Autodesk Inventor part; units mm, degrees
ref_plane "YZ Plane" through (0, 0, 0) normal (1, 0, 0) x (0, 1, 0)
ref_plane "XZ Plane" through (0, 0, 0) normal (0, 1, 0) x (-1, 0, 0)
ref_plane "XY Plane" through (0, 0, 0) normal (0, 0, 1) x (1, 0, 0)
sketch "Sketch1" plane through (0, 0, 0) normal (0, 0, 1) x (1, 0, 0)
  line L0 (-137.16, 0) -> (22.86, 0)
  line L1 (0, -160.02) -> (0, 160.02)
  arc A0 (0, 114.3) -> (0, -114.3) centre (0, 0) ccw
  arc A1 (0, 111.125) -> (0, -111.125) centre (0, 0) ccw
  line L2 (0, 111.125) -> (0, 114.3)
  line L3 (0, -114.3) -> (0, -111.125)
  dimension "d6" = 3.175
  dimension "d7" = 228.6
revolve "Revolution1" add sketch "Sketch1" angle 180 about axis through (0, -10, 0) along (0, 1, 0) contours A0 L1 A1 L0 | L0 A1 L1 A0
sketch "Sketch2" plane through (0, 0, 0) normal (0, 0, -1) x (-1, 0, 0)
  circle A0 centre (0, 0) radius 114.3
  line L0 (-6.35, 114.1235) -> (-6.35, 6.4165)
  line L1 (-6.35, 6.4165) -> (-114.1198, 6.4165)
  line L2 (160.02, 0) -> (-160.02, 0)
  line L3 (0, -160.02) -> (0, 160.02)
  line L4 (-114.3, 0.0665) -> (114.3, 0.0665) construction
  dimension "d2" = 6.35
  dimension "d3" = 6.35
extrude "Extrusion1" cut sketch "Sketch2" against normal through all contours L0 L1 A0
mirror "Mirror1" about plane through (0, 0, 0) normal (0, 1, 0) of "Extrusion1"
mirror "Mirror2" about plane through (0, 0, 0) normal (1, 0, 0) of "Extrusion1", "Mirror1"
properties part number "shell model"
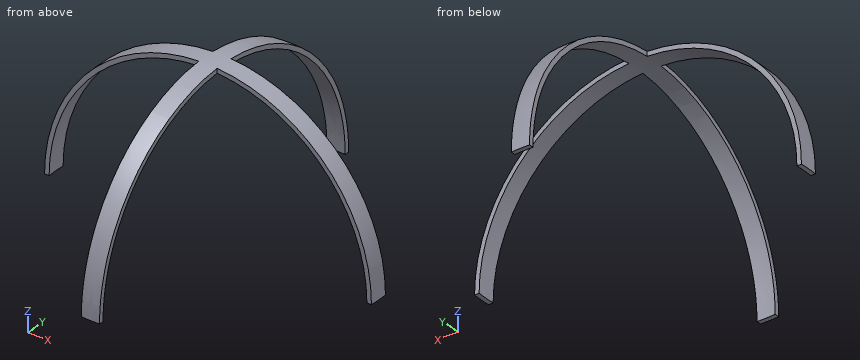
CAD build for the part. Positions are in the model's coordinates, mm. Round coordinates to 2 decimals unless told otherwise and drop trailing zeros. Write each loop counter-clockwise with the first axis right and the second up, starting at its lowest first coordinate (ties: lowest second). Pieces come first, ordered by that corner, then holes. Notation, with made-up numbers: (73, 44.25) -> (123, 44.25) arc R31 cw to (123, 73.25) -> close; hole circle Ø10 at (68.5, 52). An arc over 180 degrees is marked (long way). Answer in a Markdown table with one row per item. Add a question column.
Item 1: Saw through at C-C, the plane x = -53. Write the cut outline in (y, z).
Item 2: Drop flat-ended pins along their axis: pin 1 Ø10 at (y, z) = (-10.5, 19) entering from +X; pin 2 Ø8 at (x, y) = (5.5, -67.5) entering from -Z. Give the stop position or say it passes through.
Item 3: Drill centre lines: line 1 (X direction, y = 76.5, z = 81.5); line 2 (Z direction, x = 5, y = 20.5); line 3 (Z direction, x = 24.5, y = -5.5). Where is each one in solid material? Low to high. Write a range as from..to.
Item 4: Saw through at D-D, the plane y = 98. Write the cut outline in (x, z).
Item 5: Saw through at B-B, the plane z = 92.5. Write the cut outline in (x, y).
Item 6: Saw through at A-A, the plane z = 79. Write the cut outline in (x, y), then the cut area to 3 significant figures.
Findings below:
| question | item | result |
|---|---|---|
| 1 | outline | (-6.42, 97.46) arc R97.67 cw to (6.42, 97.46) -> (6.42, 101.07) arc R101.27 ccw to (-6.42, 101.07) -> close |
| 2 | pin 1 | stops at x = 112.98 |
| 2 | pin 2 | stops at z = 84.88 |
| 3 | line 1 | x = -6.35..6.35 |
| 3 | line 2 | z = 109.1..112.34 |
| 3 | line 3 | z = 108.25..111.51 |
| 4 | outline | (-6.35, 52) arc R52.39 cw to (6.35, 52) -> (6.35, 58.48) arc R58.83 ccw to (-6.35, 58.48) -> close |
| 5 | outline | (-66.84, -6.42) -> (-61.25, -6.42) arc R61.58 cw to (-61.25, 6.42) -> (-66.84, 6.42) arc R67.14 ccw to start; (-6.35, -66.84) arc R67.14 ccw to (6.35, -66.84) -> (6.35, -61.26) arc R61.58 cw to (-6.35, -61.26) -> close; (-6.35, 61.26) arc R61.58 cw to (6.35, 61.26) -> (6.35, 66.84) arc R67.14 ccw to (-6.35, 66.84) -> close; (61.25, -6.42) -> (66.84, -6.42) arc R67.14 ccw to (66.84, 6.42) -> (61.25, 6.42) arc R61.58 cw to start |
| 6 | outline | (-82.35, -6.42) -> (-77.89, -6.42) arc R78.15 cw to (-77.89, 6.42) -> (-82.35, 6.42) arc R82.6 ccw to start; (-6.35, -82.36) arc R82.6 ccw to (6.35, -82.36) -> (6.35, -77.89) arc R78.15 cw to (-6.35, -77.89) -> close; (-6.35, 77.89) arc R78.15 cw to (6.35, 77.89) -> (6.35, 82.36) arc R82.6 ccw to (-6.35, 82.36) -> close; (77.89, -6.42) -> (82.35, -6.42) arc R82.6 ccw to (82.35, 6.42) -> (77.89, 6.42) arc R78.15 cw to start |
| 6 | area | 228 mm^2 |
